from build123d import *

# Parameters (mm, degrees)
F0_R     = 11.5
F1_DEPTH = 1
F2_R     = 5.75
F3_DEPTH = 1
F4_R     = 4
F5_DEPTH = 7
F6_R     = 3
F7_DEPTH = 7
F8_SIZE  = 0.5


with BuildPart() as f1:
    # F0 (on Top) → F1 (new body)
    with BuildSketch(Plane.XY):
        Circle(F0_R)
    extrude(amount=F1_DEPTH)

    # F2 (on face) → F3 (join)
    with BuildSketch(Plane.XY.offset(1)):
        Circle(F2_R)
    extrude(amount=F3_DEPTH)

    # F4 (on face) → F5 (join)
    with BuildSketch(Plane.XY.offset(2)):
        Circle(F4_R)
    extrude(amount=F5_DEPTH)

    # F6 (on face) → F7 (cut)
    with BuildSketch(Plane.XY.offset(9)):
        Circle(F6_R)
    extrude(amount=-F7_DEPTH, mode=Mode.SUBTRACT)

    # F8
    f8_edges = [f1.edges().sort_by_distance(p)[0] for p in [
        (-11.5, 0, 1),
    ]]
    chamfer(f8_edges, length=F8_SIZE)


solid = f1.part
For this review, take the finished solid that the model builds, in its own axes (mm). A direction names the side the tool comes from. Coordinates: 2 decimals unless noted, no trailing zeros. Order: outer loops, then holes, each group sorted by start corner. A loop starts at its lowest first (then second) coordinate and runs counter-clockwise, first axis right, second up. Notation, with made-up numbers: (5, -32) -> (17, -32) arc R23 cw to (17, -22) -> close; hole circle Ø10 at (77.25, 43.5). An arc over 180 degrees is marked (long way). Return JSON: item names as keys, results as strings.
1. For pin 1 Ø6 at (x, y) = (-7.5, 9) entering from +Z; pin 2 Ø5 at (y, z) = (0.5, 6) entering from +X, all flat-tipped, find the tip position at first contact; note any pin that passes through.
Answer block:
{"pin 1": "z = 1", "pin 2": "x = 4"}
2. The part is to be moulded in two halves that separate along Y. For faces 3 (the cylindrical face through (-0.75, 5.7, 1.49)), 4 (the flat face through (0, 0, 2)), 5 (the flat face through (5, -5, 1)), say which applies: +Y half, -Y half, draft (parallel to the pull), parting line (faces both ways), or undercut.
Answer block:
{"face 3": "parting line", "face 4": "undercut", "face 5": "draft"}
3. We need section B-B on z = 8.5. Write out the cut boundary in (x, y).
Answer block:
{"outline": "circle Ø8 at (0, 0); hole circle Ø6 at (0, 0)"}
4. For line 1 (Y direction, x = 0, z = 7.5); line 2 (Z direction, x = -3, y = -9); line 3 (Z direction, x = 1.5, y = -1.5), list the stretches that pass through material, from the lowest coordinate up. Write a range as from..to.
Answer block:
{"line 1": "-4..-3, 3..4", "line 2": "0..1", "line 3": "0..2"}
5. Machinability: for faces 1 (the flat face through (1, 3, 9)), 2 (the flat face through (2, -4, 2)), which of the approach directions +Z, -Z, +X, -X, +Y, -Y give a long, thin tool a straight path to every point of the face, cutting with its end or side? Answer none if there is none.
Answer block:
{"face 1": "+Z, +X, -X, +Y, -Y", "face 2": "+Z"}
6. We need section A-A on x = 0. Write out the cut boundary in (y, z).
Answer block:
{"outline": "(-11.5, 0) -> (11.5, 0) -> (11.5, 0.5) -> (11, 1) -> (5.75, 1) -> (5.75, 2) -> (4, 2) -> (4, 9) -> (3, 9) -> (3, 2) -> (-3, 2) -> (-3, 9) -> (-4, 9) -> (-4, 2) -> (-5.75, 2) -> (-5.75, 1) -> (-11, 1) -> (-11.5, 0.5) -> close"}
